Input: part model. Units: mm. Frame: model coordinates. A direction names the side the tool comes from. Coordinates: 2 decimals unless noted, no trailing zeros. Write each loop counter-clockwise with the first axis right and the second up, starting at its lowest first coordinate (ties: lowest second). Pieces come first, ordered by that corner, then holes.
1) Pin query (flat end, axial travel): pin 1 Ø1 at (y, z) = (21, 36.5) entering from -X; pin 2 Ø8 at (x, y) = (-43, 5.5) entering from -Z; pin 3 Ø1.5 at (y, z) = (21.5, -13.5) entering from +X. Return the tip coordinate at first contact, or that it passes through.
2) Section query C-C (y = 6). Output: boundary loops of the cut face in (x, z).
3) Draft query along Z for faces 3 (the cylindrical face through (59.94, 4.93, -2.64)), 4 (the cylindrical face through (-1.08, 25.35, 4.88)), 5 (the flat face through (1, 0, -12)). Return one class per face: pulls with the +Z half, pulls with the -Z half, needs draft (parallel to the pull), parting line crosses it, or undercut.
4) Section query A-A (x = 0). Output: boundary loops of the cut face in (y, z), then the cut area to 3 significant figures.
5) Section query D-D (z = 46). Output: boundary loops of the cut face in (x, y), then the cut area to 3 significant figures.
6) Set-up query: faces 1 (the flat face through (-1, 50, 12)), 2 (the flat face through (23, 10, 45)). Return all of +Z, -Z, +X, -X, +Y, -Y with unobstructed straight access to the full face (end or side cutting, diameter ignored); none if empty.
7) Section query B-B (z = 0). Output: boundary loops of the cut face in (x, y).
8) Line query: L1, parallel to Y at x = 31, z = -49; L2, parallel to Z at x = 0, y = 22. Output: solid intervals per line, ascending.
Autodesk Inventor part; units mm, degrees
ref_plane "YZ Plane" through (0, 0, 0) normal (1, 0, 0) x (0, 1, 0)
ref_plane "XZ Plane" through (0, 0, 0) normal (0, 1, 0) x (-1, 0, 0)
ref_plane "XY Plane" through (0, 0, 0) normal (0, 0, 1) x (1, 0, 0)
sketch "Sketch1" plane through (0, 0, 0) normal (0, 1, 0) x (-1, 0, 0)
  circle A0 centre (0, 0) radius 60
  dimension "d0" = 120
extrude "Extrusion1" add sketch "Sketch1" along normal blind 10
sketch "Sketch2" plane through (0, 10, 0) normal (0, 1, 0) x (1, 0, 0)
  circle A0 centre (0, 0) radius 50
  dimension "d3" = 100
extrude "Extrusion2" add sketch "Sketch2" along normal blind 30
sketch "Sketch3" plane through (0, 40, 0) normal (0, 1, 0) x (1, 0, 0)
  circle A0 centre (0, 0) radius 60
  circle A1 centre (0, 0) radius 5
  dimension "d6" = 120
  dimension "d9" = 10
extrude "Extrusion3" add sketch "Sketch3" along normal blind 10 contours A0 | A1
sketch "Sketch5" plane through (0, 50, 0) normal (0, 1, 0) x (1, 0, 0)
  circle A0 centre (0, 0) radius 5
  dimension "d10" = 10
extrude "Extrusion4" cut sketch "Sketch5" against normal through all
properties part number "drivepulley"
Answer:
1. pin 1: stops at x = -34.7
1. pin 2: stops at z = -45.6
1. pin 3: stops at x = 48.35
2. outline: circle Ø120 at (0, 0); hole circle Ø10 at (0, 0)
3. face 3: parting line crosses it
3. face 4: undercut
3. face 5: needs draft
4. outline: (0, -60) - (10, -60) - (10, -50) - (40, -50) - (40, -60) - (50, -60) - (50, -5) - (0, -5) - close; (0, 5) - (50, 5) - (50, 60) - (40, 60) - (40, 50) - (10, 50) - (10, 60) - (0, 60) - close
4. area: 4,900 mm2
5. outline: (-38.52, 0) - (38.52, 0) - (38.52, 10) - (19.6, 10) - (19.6, 40) - (38.52, 40) - (38.52, 50) - (-38.52, 50) - (-38.52, 40) - (-19.6, 40) - (-19.6, 10) - (-38.52, 10) - close
5. area: 2,720 mm2
6. face 1: +Z, -Z, +X, -X, +Y
6. face 2: none
7. outline: (-60, 0) - (-5, 0) - (-5, 50) - (-60, 50) - (-60, 40) - (-50, 40) - (-50, 10) - (-60, 10) - close; (5, 0) - (60, 0) - (60, 10) - (50, 10) - (50, 40) - (60, 40) - (60, 50) - (5, 50) - close
8. L1: y = 0 to 10, 40 to 50
8. L2: z = -50 to -5, 5 to 50
